Part model, mm, in its own coordinate system. Round coordinates to 2 decimals unless told otherwise and drop trailing zeros. Loops run counter-clockwise (first coordinate to the right, second up) from the corner with the lowest first, then second, coordinate; pieces in that order, holes last. Notation, with made-up numbers: (2.25, 53) -> (32.25, 53) arc R18 ccw to (32.25, 74) -> close; hole circle Ø7 at (88.5, 34). An arc over 180 degrees is marked (long way). Use a Markdown table: item, result. Add a question column.
Item 1: Probe line 1 (Y direction, x = 103, z = 2.9); line 2 (Y direction, x = 98.5, z = 3). List the from-to ranges inside material, lowest first. Write a range as [from, to].
Item 2: Flat gauge pin, fed straight in: pin 1 (0.8 mm diameter, centred on x = 4.5, y = 2, fed in from +Z) (3 decimals). Where does the tip first touch, or does it go through?
Item 3: Cut at A-A, the plane x = 100. List the corners of the cut face in (y, z) (3 decimals), plus the area to 3 significant figures.
Item 4: Two-plate mould, pull along X, no slides. Class faces 1 (the face through (100.269, 12.748, 1.61)), 2 (the face through (99, 101, 3.175)): pulls with the +X half, pulls with the -X half, needs draft (parallel to the pull), parting line crosses it, or undercut.
```python
from build123d import *

# Parameters (mm, degrees)
SKETCH1_W           = 200
SKETCH1_H           = 200
BOSS_EXTRUDE1_DEPTH = 3.175
SKETCH5_W           = 200
SKETCH5_H           = 200
SKETCH5_W_2         = 199.8984
SKETCH5_H_2         = 199.8984
CUT_EXTRUDE2_DEPTH  = 283.860532109
CUT_EXTRUDE1_DEPTH  = 3.175
FILLET1_R           = 0.79375
SKETCH6_R           = 0.79375
CUT_EXTRUDE3_DEPTH  = 1.27
LPATTERN1_COUNT     = 4
LPATTERN1_PITCH     = 2.54


with BuildPart() as part:
    # Sketch1 → Boss-Extrude1 (new body)
    with BuildSketch(Plane.XY):
        with Locations((100, 100)):
            Rectangle(SKETCH1_W, SKETCH1_H)
    extrude(amount=BOSS_EXTRUDE1_DEPTH)

    # Sketch5 → Cut-Extrude2 (cut, through all)
    with BuildSketch(Plane.XY.offset(3.175)):
        with Locations((100, 100)):
            Rectangle(SKETCH5_W, SKETCH5_H)
        with Locations((100, 100)):
            Rectangle(SKETCH5_W_2, SKETCH5_H_2, mode=Mode.SUBTRACT)
    extrude(amount=-CUT_EXTRUDE2_DEPTH, mode=Mode.SUBTRACT)

    # Sketch2 → Cut-Extrude1 (cut)
    with BuildSketch(Plane.XY.offset(3.175)):
        with BuildLine():
            Line((87.3, 0.0508), (112.7, 0.0508))
            ThreePointArc((112.7, 0.0508), (100, 12.7508), (87.3, 0.0508))
        make_face()
    extrude(amount=-CUT_EXTRUDE1_DEPTH, mode=Mode.SUBTRACT)

    # Fillet1
    fillet1_edges = [part.edges().sort_by_distance(p)[0] for p in [
        (87.3, 0.0508, 1.5875),
        (112.7, 0.0508, 1.5875),
    ]]
    fillet(fillet1_edges, radius=FILLET1_R)

    # Sketch6 → Cut-Extrude3 (cut)
    with BuildSketch(Plane.XY.offset(3.175)):
        with Locations((2.0828, 2.0828)):
            Circle(SKETCH6_R)
    cut_extrude3 = extrude(amount=-CUT_EXTRUDE3_DEPTH, mode=Mode.SUBTRACT)

    # LPattern1: Cut-Extrude3 ×4
    with Locations(*[(i * LPATTERN1_PITCH, 0, 0) for i in range(1, LPATTERN1_COUNT)]):
        add(cut_extrude3, mode=Mode.SUBTRACT)


solid = part.part
```
A:
| question | item | result |
|---|---|---|
| 1 | line 1 | y = [12.39, 199.95] |
| 1 | line 2 | y = [12.66, 199.95] |
| 2 | pin 1 | stops at z = 1.905 |
| 3 | outline | (12.751, 0) -> (199.949, 0) -> (199.949, 3.175) -> (12.751, 3.175) -> close |
| 3 | area | 594 mm^2 |
| 4 | face 1 | undercut |
| 4 | face 2 | needs draft |
